from build123d import *

# Parameters (mm, degrees)
SKETCH1_R           = 28.4
BOSS_EXTRUDE1_DEPTH = 3
SKETCH2_R           = 11
BOSS_EXTRUDE2_DEPTH = 20
SKETCH3_R           = 3
CUT_EXTRUDE1_DEPTH  = 24
SKETCH4_R           = 2
CUT_EXTRUDE2_DEPTH  = 15
CHAMFER1_SIZE       = 1
SKETCH5_R           = 2
CUT_EXTRUDE5_DEPTH  = 4.0000001
CIRPATTERN2_COUNT   = 12


with BuildPart() as part:
    # Sketch1 → Boss-Extrude1 (new body)
    with BuildSketch(Plane.XY):
        Circle(SKETCH1_R)
    extrude(amount=BOSS_EXTRUDE1_DEPTH)

    # Sketch2 → Boss-Extrude2 (add)
    with BuildSketch(Plane.XY.offset(3)):
        Circle(SKETCH2_R)
    extrude(amount=BOSS_EXTRUDE2_DEPTH)

    # Sketch3 → Cut-Extrude1 (cut, through all)
    with BuildSketch(Plane.XY.offset(23)):
        Circle(SKETCH3_R)
    extrude(amount=-CUT_EXTRUDE1_DEPTH, mode=Mode.SUBTRACT)

    # Sketch4 → Cut-Extrude2 (cut)
    with BuildSketch(Plane(origin=(0, 0, 0), x_dir=(1, 0, 0), z_dir=(0, 1, 0))):
        with Locations((0, -15)):
            Circle(SKETCH4_R)
    extrude(amount=-CUT_EXTRUDE2_DEPTH, mode=Mode.SUBTRACT)

    # Chamfer1
    chamfer1_edges = [part.edges().sort_by_distance(p)[0] for p in [
        (-11, 0, 3),
        (-11, 0, 23),
    ]]
    chamfer(chamfer1_edges, length=CHAMFER1_SIZE)

    # Sketch5 → Cut-Extrude5 (cut, through all)
    with BuildSketch(Plane.XY.offset(3)):
        with Locations((11.9, 20.61140461)):
            Circle(SKETCH5_R)
    cut_extrude5 = extrude(amount=-CUT_EXTRUDE5_DEPTH, mode=Mode.SUBTRACT)

    # CirPattern2: Cut-Extrude5 ×12 about axis
    cirpattern2_axis = Axis((0, 0, 0), (0, 0, 1))
    for i in range(1, CIRPATTERN2_COUNT):
        add(cut_extrude5.rotate(cirpattern2_axis, i * 360 / CIRPATTERN2_COUNT), mode=Mode.SUBTRACT)


solid = part.part
Geometry: final body of the model. Coordinates: model frame, mm. A direction names the side the tool comes from. Give positions to 0.01 mm unless a question says otherwise; leave off trailing zeros. Write each loop counter-clockwise with the first axis right and the second up, starting at its lowest first coordinate (ties: lowest second). Pieces come first, ordered by that corner, then holes. Notation, with made-up numbers: M 18.5,72 L 64.5,72 A33 cw 64.5,107 Z; hole C -18,41.5 d8. An arc over 180 degrees is marked long. Answer in a Markdown table with one row per item. Add a question column.
(1) Section B-B on x = -23.8. Return loops of the section in (y, z).
(2) Ray query, line 1 (Y direction, x = -11.9, z = 1.8); line 2 (Z direction, x = 10, y = 12.5); line 3 (Y direction, x = -23.8, z = 2.1). Return the intervals inside material, ascending.
(3) First-contact query: pin 1 (5 mm diameter, centred on x = 11.9, y = 20.61, fed in from +Z); pin 2 (2 mm diameter, centred on x = -10.5, z = 17.5, fed in from +Y); pin 3 (4.5 mm diameter, centred on x = 0, z = 15, fed in from +Y); pin 4 (6.5 mm diameter, centred on x = 23.8, y = 0, fed in from -Z). Flat tips, straight axial feed; report the tip coordinate or a pass-through.
(4) Mould query, pull axis X, two halves, no side actions, for faces 3 (the cylindrical face through (-2, -7, 15)), 4 (the flat face through (2.1, 2.4, 23)), 5 (the cylindrical face through (-2.38, -10.74, 12.87)), 6 (the cylindrical face through (-18.925, -12.975, 1.521)). Classes: +X half, -X half, draft (parallel to the pull), parting line (faces both ways), or undercut.
(5) Section C-C on y = -13. Return loops of the section in (x, z).
(6) Section A-A on y = 0. Return loops of the section in (x, z).
(7) Reachability of faces 1 (the flat face through (-0.4, -12.2, 3)), 2 (the cylindrical face through (19.85, -13.75, 1.52)) from +Z, -Z, +X, -X, +Y, -Y: full face, straight path, thin tool, end or side. Return the list, or none.
Result set:
| question | item | result |
|---|---|---|
| 1 | outline | M -15.5,0 L -2,0 L -2,3 L -15.5,3 Z; M 2,0 L 15.5,0 L 15.5,3 L 2,3 Z |
| 2 | line 1 | y = -25.79 to -22.61, -18.61 to 18.61, 22.61 to 25.79 |
| 2 | line 2 | z = 0 to 3 |
| 2 | line 3 | y = -15.5 to -2, 2 to 15.5 |
| 3 | pin 1 | stops at z = 3 |
| 3 | pin 2 | stops at y = 5.55 |
| 3 | pin 3 | stops at y = 11 |
| 3 | pin 4 | stops at z = 0 |
| 4 | face 3 | undercut |
| 4 | face 4 | draft |
| 4 | face 5 | parting line |
| 4 | face 6 | undercut |
| 5 | outline | M -25.25,0 L -22.28,0 L -22.28,3 L -25.25,3 Z; M -18.94,0 L 18.94,0 L 18.94,3 L -18.94,3 Z; M 22.28,0 L 25.25,0 L 25.25,3 L 22.28,3 Z |
| 6 | outline | M -28.4,0 L -25.8,0 L -25.8,3 L -28.4,3 Z; M -21.8,0 L -3,0 L -3,23 L -10,23 L -11,22 L -11,4 L -12,3 L -21.8,3 Z; M 3,0 L 21.8,0 L 21.8,3 L 12,3 L 11,4 L 11,22 L 10,23 L 3,23 Z; M 25.8,0 L 28.4,0 L 28.4,3 L 25.8,3 Z |
| 7 | face 1 | +Z |
| 7 | face 2 | +Z, -Z |
